Input: part model. Units: mm. Frame: model coordinates. Give positions to 0.01 mm unless a question says otherwise; leave off trailing zeros. Loops run counter-clockwise (first coordinate to the right, second up) from the corner with the lowest first, then second, coordinate; pieces in that order, holes last. Notation, with made-up numbers: (86, -39) - (97, -39) arc R30 ccw to (97, -4) - close; hole circle Ø11 at (22, 84.5). An arc over 180 degrees is marked (long way). Answer as a JSON object with one key per item and string values. Group by question number.
(1) Mould query, pull axis Y, two halves, no side actions, for faces 1 (the cylindrical face through (-59.474, -0.481, 2.465)), 2 (the cylindrical face through (36.69, -57.55, 2.46)), 3 (the flat face through (35, 41, 0)), 4 (the cylindrical face through (-11.598, 52.228, 2.465)). Classes: +Y half, -Y half, draft (parallel to the pull), parting line (faces both ways), or undercut.
(2) Section query D-D (x = 61). Return loops of the section in (y, z), plus the area to 3 significant figures.
(3) Section query C-C (z = 3.55). Return loops of the section in (x, y).
(4) Pin query (flat end, axial travel): P1, Ø8, axis at x = 33, y = -34.5, coming from the +Z side; P2, Ø3, axis at x = -2, z = 1.5, coming from the -Y side. Return the tip coordinate at first contact, or that it passes through.
(5) Material intervals for L1, parallel to Y at x = 0, z = 2.5; L2, parallel to Y at x = -0.5, z = 0.4; L3, parallel to Y at x = 46, z = 2.1, sorted ascending.
(6) Section query A-A (x = 0). Return loops of the section in (y, z).
Autodesk Inventor part; units mm, degrees
ref_plane "YZ Plane" through (0, 0, 0) normal (1, 0, 0) x (0, 1, 0)
ref_plane "XZ Plane" through (0, 0, 0) normal (0, 1, 0) x (-1, 0, 0)
ref_plane "XY Plane" through (0, 0, 0) normal (0, 0, 1) x (1, 0, 0)
sketch "스케치1" plane through (0, 0, 0) normal (0, 0, 1) x (1, 0, 0)
  circle A0 centre (0, 0) radius 68.25
  circle A1 centre (0, 0) radius 53.5
  circle A2 centre (0, 0) radius 61 construction
  circle A3 centre (0, 61) radius 1.6
  circle A4 centre (-61, 0) radius 1.6
  circle A5 centre (0, -61) radius 1.6
  circle A6 centre (61, 0) radius 1.6
  dimension "d2" = 122
  dimension "d0" = 136.5
  dimension "d1" = 107
  dimension "d3" = 3.2
  dimension "d6" = 360
extrude "돌출1" add sketch "스케치1" along normal blind 5
properties part number "아크릴 빛번짐 고정용"
Recorded:
{
 "1": {"face 1": "undercut", "face 2": "parting line", "face 3": "draft", "face 4": "undercut"},
 "2": {"outline": "(-30.61, 0) - (-1.6, 0) - (-1.6, 5) - (-30.61, 5) - close; (1.6, 0) - (30.61, 0) - (30.61, 5) - (1.6, 5) - close", "area": "290 mm^2"},
 "3": {"outline": "circle Ø136.5 at (0, 0); hole circle Ø3.2 at (-61, 0); hole circle Ø107 at (0, 0); hole circle Ø3.2 at (0, -61); hole circle Ø3.2 at (0, 61); hole circle Ø3.2 at (61, 0)"},
 "4": {"P1": "passes through", "P2": "stops at y = -68.25"},
 "5": {"L1": "y = -68.25 to -62.6, -59.4 to -53.5, 53.5 to 59.4, 62.6 to 68.25", "L2": "y = -68.25 to -62.52, -59.48 to -53.5, 53.5 to 59.48, 62.52 to 68.25", "L3": "y = -50.42 to -27.32, 27.32 to 50.42"},
 "6": {"outline": "(-68.25, 0) - (-62.6, 0) - (-62.6, 5) - (-68.25, 5) - close; (-59.4, 0) - (-53.5, 0) - (-53.5, 5) - (-59.4, 5) - close; (53.5, 0) - (59.4, 0) - (59.4, 5) - (53.5, 5) - close; (62.6, 0) - (68.25, 0) - (68.25, 5) - (62.6, 5) - close"}
}
